The figure shows three views and two pictorial views of one solid part (mm, origin at its lowest corner). Answer the questions. A direction names the side the tool comes from. Coordinates: 2 decimals unless noted, no trailing zeros. Order: outer loops, then holes, each group sorted by start corner. A loop starts at its lowest first (then second) coordinate and runs counter-clockwise, first axis right, second up.
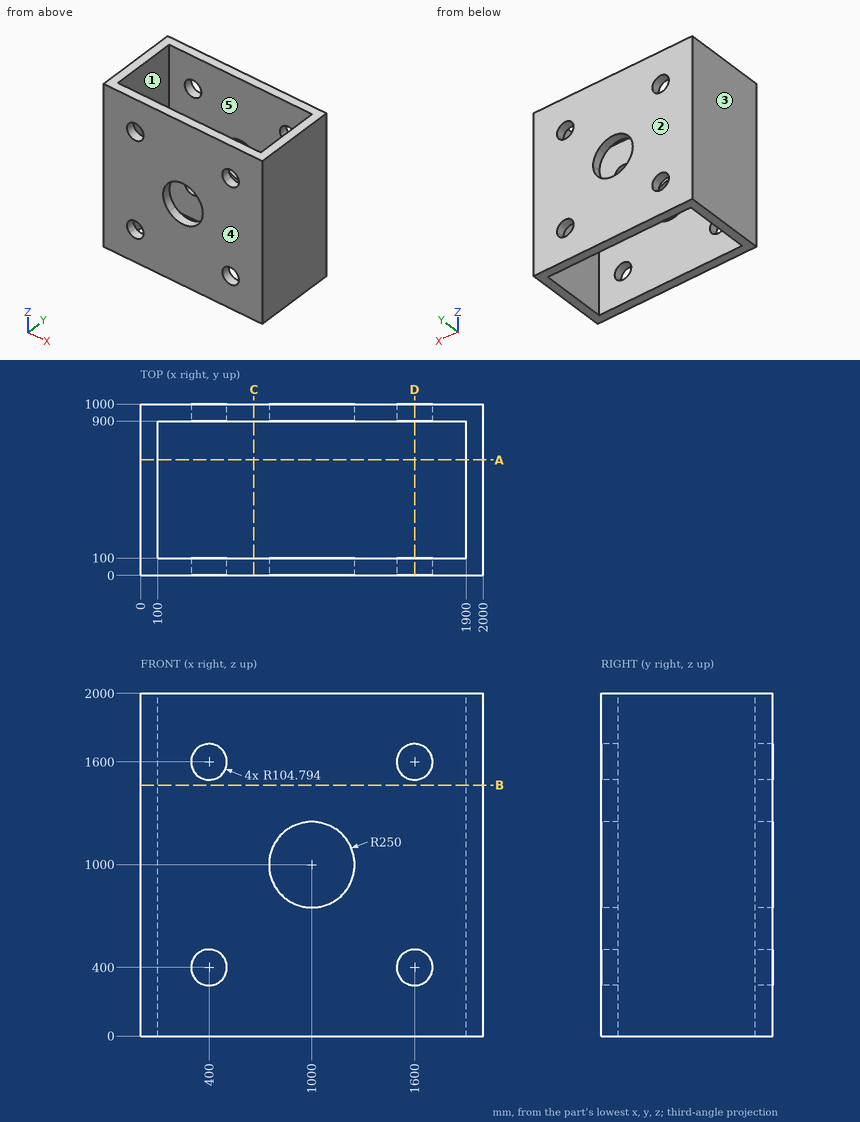
Q1. The part is cut by section B-B, the plane z = 1464. Determine the outline of the cut face in (x, y).
Q2. The part is cut by section D-D, the plane x = 1600. Determine the outline of the cut face in (y, z).
Q3. Straight lines are drawn through the part: L1, parallel to Y at x = 850, z = 1437; L2, parallel to X at y = 357, z = 724.5; L3, parallel to Z at x = 1695.5, y = 43 (1 decimal). For each, find the intervals that lie inside material, in ascending order.
Q4. Which of the six approach directions +Z, -Z, +X, -X, +Y, -Y give full straight-line access (tool end or side, diameter ignored) to the marked faces 4 and 5?
Q5. The part is cut by section A-A, the plane y = 674. Determine the outline of the cut face in (x, z), then the cut area to 3 significant figures.
Q6. Determine the mould class of the marked faces 1, 2 and 3 for opening direction Y: +Y half, -Y half, draft (parallel to the pull), parting line (faces both ways), or undercut.
Q7. The part is cut by section C-C, the plane x = 662. Determine the outline of the cut face in (y, z), then the cut area to 3 significant figures.
Computed values:
1. outline: (0, 0) - (2000, 0) - (2000, 1000) - (0, 1000) - close; hole (100, 100) - (1900, 100) - (1900, 900) - (100, 900) - close
2. outline: (0, 0) - (100, 0) - (100, 295.21) - (0, 295.21) - close; (0, 504.79) - (100, 504.79) - (100, 1495.21) - (0, 1495.21) - close; (0, 1704.79) - (100, 1704.79) - (100, 2000) - (0, 2000) - close; (900, 0) - (1000, 0) - (1000, 295.21) - (900, 295.21) - close; (900, 504.79) - (1000, 504.79) - (1000, 1495.21) - (900, 1495.21) - close; (900, 1704.79) - (1000, 1704.79) - (1000, 2000) - (900, 2000) - close
3. L1: y = 0 to 100, 900 to 1000
3. L2: x = 0 to 100, 1900 to 2000
3. L3: z = 0 to 356.9, 443.1 to 1556.9, 1643.1 to 2000
4. face 4: +Z, -Z, +X, -X, -Y
4. face 5: +Z, -Z
5. outline: (0, 0) - (100, 0) - (100, 2000) - (0, 2000) - close; (1900, 0) - (2000, 0) - (2000, 2000) - (1900, 2000) - close
5. area: 400,000 mm2
6. face 1: undercut
6. face 2: +Y half
6. face 3: draft
7. outline: (0, 0) - (100, 0) - (100, 2000) - (0, 2000) - close; (900, 0) - (1000, 0) - (1000, 2000) - (900, 2000) - close
7. area: 400,000 mm2
